from build123d import *

# Parameters (mm, degrees)
F0_R     = 0.32131
F0_W     = 15.24
F0_H     = 12.192
F1_DEPTH = 0.762
F2_DEPTH = 2.286


with BuildPart() as f1:
    # F0 (on Top) → F1 (new body)
    with BuildSketch(Plane.XY):
        with BuildLine():
            Line((12.065, -8.001), (12.065, 8.001))
            Line((12.065, 8.001), (10.836146, 8.001))
            ThreePointArc((10.836146, 8.001), (10.541, 7.80669), (10.245854, 8.001))
            Line((10.245854, 8.001), (8.804146, 8.001))
            ThreePointArc((8.804146, 8.001), (8.509, 7.80669), (8.213854, 8.001))
            Line((8.213854, 8.001), (6.772146, 8.001))
            ThreePointArc((6.772146, 8.001), (6.477, 7.80669), (6.181854, 8.001))
            Line((6.181854, 8.001), (4.740146, 8.001))
            ThreePointArc((4.740146, 8.001), (4.445, 7.80669), (4.149854, 8.001))
            Line((4.149854, 8.001), (2.708146, 8.001))
            ThreePointArc((2.708146, 8.001), (2.413, 7.80669), (2.117854, 8.001))
            Line((2.117854, 8.001), (0.676146, 8.001))
            ThreePointArc((0.676146, 8.001), (0.381, 7.80669), (0.085854, 8.001))
            Line((0.085854, 8.001), (-1.355854, 8.001))
            ThreePointArc((-1.355854, 8.001), (-1.651, 7.80669), (-1.946146, 8.001))
            Line((-1.946146, 8.001), (-3.387854, 8.001))
            ThreePointArc((-3.387854, 8.001), (-3.683, 7.80669), (-3.978146, 8.001))
            Line((-3.978146, 8.001), (-12.065, 8.001))
            Line((-12.065, 8.001), (-12.065, -8.001))
            Line((-12.065, -8.001), (-3.992706, -8.001))
            ThreePointArc((-3.992706, -8.001), (-3.69756, -7.80669), (-3.402414, -8.001))
            Line((-3.402414, -8.001), (-1.958626, -8.001))
            ThreePointArc((-1.958626, -8.001), (-1.66348, -7.80669), (-1.368334, -8.001))
            Line((-1.368334, -8.001), (0.075454, -8.001))
            ThreePointArc((0.075454, -8.001), (0.3706, -7.80669), (0.665746, -8.001))
            Line((0.665746, -8.001), (2.109534, -8.001))
            ThreePointArc((2.109534, -8.001), (2.40468, -7.80669), (2.699826, -8.001))
            Line((2.699826, -8.001), (4.143614, -8.001))
            ThreePointArc((4.143614, -8.001), (4.43876, -7.80669), (4.733906, -8.001))
            Line((4.733906, -8.001), (6.177694, -8.001))
            ThreePointArc((6.177694, -8.001), (6.47284, -7.80669), (6.767986, -8.001))
            Line((6.767986, -8.001), (8.211774, -8.001))
            ThreePointArc((8.211774, -8.001), (8.50692, -7.80669), (8.802066, -8.001))
            Line((8.802066, -8.001), (10.245854, -8.001))
            ThreePointArc((10.245854, -8.001), (10.541, -7.80669), (10.836146, -8.001))
            Line((10.836146, -8.001), (12.065, -8.001))
        make_face()
        with Locations((-3.69721, -7.239)):
            Circle(F0_R, mode=Mode.SUBTRACT)
        with Locations((-1.66318, -7.239)):
            Circle(F0_R, mode=Mode.SUBTRACT)
        with Locations((0.37085, -7.239)):
            Circle(F0_R, mode=Mode.SUBTRACT)
        with Locations((2.40488, -7.239)):
            Circle(F0_R, mode=Mode.SUBTRACT)
        with Locations((4.43891, -7.239)):
            Circle(F0_R, mode=Mode.SUBTRACT)
        with Locations((6.47294, -7.239)):
            Circle(F0_R, mode=Mode.SUBTRACT)
        with Locations((8.50697, -7.239)):
            Circle(F0_R, mode=Mode.SUBTRACT)
        with Locations((10.541, -7.239)):
            Circle(F0_R, mode=Mode.SUBTRACT)
        with Locations((-3.64905, 7.239)):
            Circle(F0_R, mode=Mode.SUBTRACT)
        with Locations((-1.6219, 7.239)):
            Circle(F0_R, mode=Mode.SUBTRACT)
        with Locations((3.429, 0)):
            Rectangle(F0_W, F0_H, mode=Mode.SUBTRACT)
        with Locations((0.40525, 7.239)):
            Circle(F0_R, mode=Mode.SUBTRACT)
        with Locations((2.4324, 7.239)):
            Circle(F0_R, mode=Mode.SUBTRACT)
        with Locations((4.45955, 7.239)):
            Circle(F0_R, mode=Mode.SUBTRACT)
        with Locations((6.4867, 7.239)):
            Circle(F0_R, mode=Mode.SUBTRACT)
        with Locations((8.51385, 7.239)):
            Circle(F0_R, mode=Mode.SUBTRACT)
        with Locations((10.541, 7.239)):
            Circle(F0_R, mode=Mode.SUBTRACT)
        with Locations((3.429, 0)):
            Rectangle(F0_W, F0_H)
    extrude(amount=-F1_DEPTH)

    # F0 (on Top) → F2 (join)
    with BuildSketch(Plane.XY):
        with Locations((3.429, 0)):
            Rectangle(F0_W, F0_H)
    extrude(amount=F2_DEPTH)


solid = f1.part
The model under review builds one solid part; all positions refer to its coordinate system, in mm. A direction names the side the tool comes from. Coordinates: 2 decimals unless noted, no trailing zeros. Write each loop counter-clockwise with the first axis right and the second up, starting at its lowest first coordinate (ties: lowest second). Pieces come first, ordered by that corner, then holes. Notation, with made-up numbers: (-39.75, 56.5) - (-12.75, 56.5) arc R22 ccw to (-12.75, 64.5) - close; hole circle Ø9 at (-19, 64.25). An arc over 180 degrees is marked (long way). Answer as CSV lines item,"result".
(1) Tool access review of faces 1 (the flat face through (-4.191, 0, 1)), 2 (the flat face through (3, -6.096, 1)), 3 (the flat face through (11.049, 0, 1)), 4 (the flat face through (3, 6.096, 1)): name each direction out of +Z, -Z, +X, -X, +Y, -Y from which nothing blocks a thin tool from reaching the whole face with its end or side.
Data:
face 1,"+Z, -X, +Y, -Y"
face 2,"+Z, +X, -X, -Y"
face 3,"+Z, +X, +Y, -Y"
face 4,"+Z, +X, -X, +Y"
(2) We need section C-C (x = 6.5). Give the boundary of the cut face in (y, z), plus the area to 3 significant figures.
Data:
outline,"(-7.81, -0.76) - (-7.56, -0.76) - (-7.56, 0) - (-7.81, 0) - close; (-6.92, -0.76) - (6.92, -0.76) - (6.92, 0) - (6.1, 0) - (6.1, 2.29) - (-6.1, 2.29) - (-6.1, 0) - (-6.92, 0) - close; (7.56, -0.76) - (7.81, -0.76) - (7.81, 0) - (7.56, 0) - close"
area,"38.8 mm2"
(3) We need section D-D (z = 0.85). Give the boundary of the cut face in (x, y).
Data:
outline,"(-4.19, -6.1) - (11.05, -6.1) - (11.05, 6.1) - (-4.19, 6.1) - close"
(4) Clearance check with flat-ended pins moving along their axes: pin 1 Ø1 at (y, z) = (-6, 1) entering from -X; pin 2 Ø1 at (y, z) = (2, 1) entering from +X; pin 3 Ø0.7 at (x, z) = (5, 1) entering from -Y. State where each tip first meets the part, or that it passes through.
Data:
pin 1,"stops at x = -4.19"
pin 2,"stops at x = 11.05"
pin 3,"stops at y = -6.1"
(5) We need section B-B (x = -0.5). Give the boundary of the cut face in (y, z).
Data:
outline,"(-8, -0.76) - (8, -0.76) - (8, 0) - (6.1, 0) - (6.1, 2.29) - (-6.1, 2.29) - (-6.1, 0) - (-8, 0) - close"
(6) We need section A-A (y = -4.25). Give the boundary of the cut face in (x, z) (3 decimals).
Data:
outline,"(-12.065, -0.762) - (12.065, -0.762) - (12.065, 0) - (11.049, 0) - (11.049, 2.286) - (-4.191, 2.286) - (-4.191, 0) - (-12.065, 0) - close"
(7) For line 1 along Z through (x, y) = (0.5, 6.5); line 2 along X through (y, z) = (-3.5, 1.2); line 3 along Y through (x, z) = (6.75, 1.8), list the stretches that pass through material, from the lowest coordinate up. Write a range as [from, to].
Data:
line 1,"z = [-0.76, 0]"
line 2,"x = [-4.19, 11.05]"
line 3,"y = [-6.1, 6.1]"
